Geometry check sheet. Reference: drawing and pictorial views, mm from the part's lowest x, y, z. Give positions to 0.01 mm unless a question says otherwise; leave off trailing zeros. Order: outer loops, then holes, each group sorted by start corner. A loop starts at its lowest first (then second) coordinate and runs counter-clockwise, first axis right, second up. Notation, with made-up numbers: (-29, 13.25) -> (-19, 13.25) arc R36 cw to (-19, 52.25) -> close; hole circle Ø10 at (59.5, -28.75). An arc over 180 degrees is marked (long way). Write each question's results on one line, items separated by ' | '. Start each with the question number.
1. Cross-section at D-D, the plane y = 23.5. Enter the section's corners in (x, z).
2. Depth check by flat-ended pin: pin 1 Ø10 at (x, y) = (49, 12) entering from -Z; pin 2 Ø4 at (y, z) = (21, 8.5) entering from -X. Enter the tip coordinate at first touch or a pass-through.
3. Material ranges on L1, parallel to Y at x = 21.4, z = 13.75; L2, parallel to Z at x = 4, y = 10; L3, parallel to Y at x = 22, z = 4.25, recorded low to high. Write a range as from..to.
4. Cross-section at C-C, the plane z = 2. Enter the section's corners in (x, y).
5. Cross-section at B-B, the plane x = 8. Enter the section's corners in (y, z).
6. Cross-section at A-A, the plane x = 21.4. Enter the section's corners in (y, z), then the cut area to 3 significant figures.
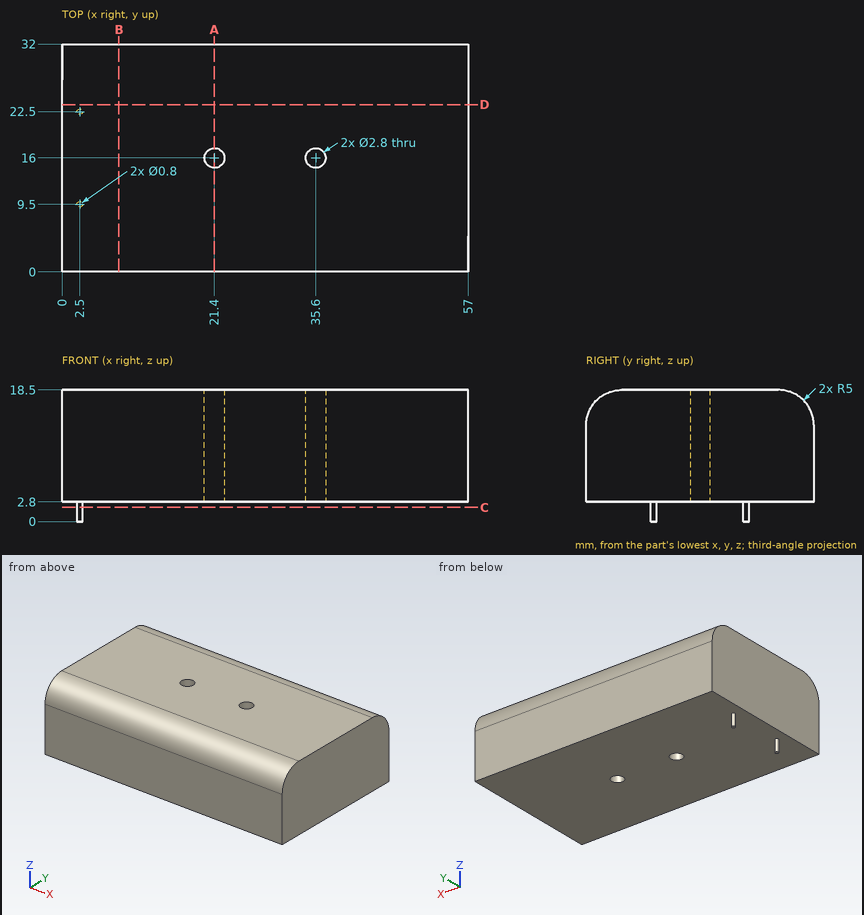
Results below:
1) outline: (0, 2.8) -> (57, 2.8) -> (57, 18.5) -> (0, 18.5) -> close
2) pin 1: stops at z = 2.8 | pin 2: stops at x = 0
3) L1: y = 0.01..14.6, 17.4..31.99 | L2: z = 2.8..18.5 | L3: y = 0..14.74, 17.26..32
4) outline: circle Ø0.8 at (2.5, 9.5); circle Ø0.8 at (2.5, 22.5)
5) outline: (0, 2.8) -> (32, 2.8) -> (32, 13.5) arc R5 ccw to (27, 18.5) -> (5, 18.5) arc R5 ccw to (0, 13.5) -> close
6) outline: (0, 2.8) -> (14.6, 2.8) -> (14.6, 18.5) -> (5, 18.5) arc R5 ccw to (0, 13.5) -> close; (17.4, 2.8) -> (32, 2.8) -> (32, 13.5) arc R5 ccw to (27, 18.5) -> (17.4, 18.5) -> close | area: 448 mm²
